Verification items for the finished model (mm, model axes). A direction names the side the tool comes from. Coordinates: 2 decimals unless noted, no trailing zeros. Order: outer loops, then holes, each group sorted by start corner. A loop starts at its lowest first (then second) coordinate and runs counter-clockwise, first axis right, second up. Notation, with made-up numbers: (55, 0) -> (112, 0) arc R26 cw to (112, 39) -> close; hole circle Ø3 at (80, 11.25). An arc over 180 degrees is marked (long way). Write item = value, one per line. Start each with the question number.
1. Go/stop test with flat-tipped pins: P1, Ø1.6, axis at x = -0.5, y = -16, coming from the +Z side; P2, Ø4, axis at x = 0, y = 0, coming from the +Z side; P3, Ø1, axis at x = -2, z = 3.5, coming from the +Y side. Record where each tip stops, or that it passes through.
2. Set-up check for faces 4 (the flat face through (-2.6, -17.5, 2.76)), 5 (the flat face through (0, -8, 4.8)), 6 (the flat face through (0, -18, 3.26)), 7 (the flat face through (-4.943, -6.509, 2.266)), 8 (the flat face through (0, -2, 2.54)): record each of +Z, -Z, +X, -X, +Y, -Y from which the full face is reachable in a straight line by a thin tool's end or side.
3. Cross-section at B-B on y = -23.5. Record the cut outline in (x, z).
4. Release check for a two-part mould opening along Y. For faces 1 (the cylindrical face through (-0.345, -1.552, 1.252)), 2 (the flat face through (-0.071, -12.448, 1.361)), 3 (the flat face through (0, -4, 0)) record: +Y half, -Y half, draft (parallel to the pull), parting line (faces both ways), or undercut.
5. Thickness scan on line 1 along X through (y, z) = (0, 2.05); line 2 along Y through (x, z) = (0, 1.45); line 3 along Y through (x, z) = (0, 0.6). Record the ranges inside material, lowest first. Write a range as from..to.
6. Cross-section at C-C on x = -3.75. Record the cut outline in (y, z).
7. Cross-section at A-A on y = 0. Record the cut outline in (x, z), plus the area to 3 significant figures.
8. Cross-section at D-D on z = 1.8. Record the cut outline in (x, y), plus the area to 3 significant figures.
from build123d import *

# Parameters (mm, degrees)
SKETCH1_W          = 10.16
SKETCH1_H          = 15.87
SKETCH1_R          = 1.59
EXTRUDE1_DEPTH     = 4.8
SKETCH2_W          = 4.533761675
SKETCH2_H          = 11.038854263
CUT_EXTRUDE1_DEPTH = 5.5
CHAMFER1_SIZE      = 1
EXTRUDE2_DEPTH     = 0.5
DRAFT1_START       = -14
DRAFT1_DEPTH       = 17.3
DRAFT1_START_2     = 3.226433484
DRAFT1_2_OUTLINE_W = 14
DRAFT1_2_OUTLINE_H = 3
DRAFT1_2_DEPTH     = 0.773566516
DRAFT2_ANGLE       = -5
DRAFT4_START       = -5.08
DRAFT4_DEPTH       = 10.16
DRAFT4_2_DEPTH     = 1.805
DRAFT4_START_2     = 3.275
DRAFT4_3_DEPTH     = 1.805
DRAFT4_START_3     = -1.805
DRAFT4_4_DEPTH     = 1.07
DRAFT4_START_4     = 0.735
DRAFT4_5_DEPTH     = 1.07
DRAFT3_ANGLE       = 5


with BuildPart() as part:
    # Sketch1 → Extrude1 (new body)
    with BuildSketch(Plane.XY):
        with Locations((0, -4.635)):
            Rectangle(SKETCH1_W, SKETCH1_H)
        Circle(SKETCH1_R, mode=Mode.SUBTRACT)
    extrude(amount=EXTRUDE1_DEPTH)

    # Sketch2 → Cut-Extrude1 (cut, symmetric)
    with BuildSketch(Plane(origin=(0, 0, 0), x_dir=(0, 0, -1), z_dir=(1, 0, 0))):
        with Locations((-4.806880837, 2.139427131)):
            Rectangle(SKETCH2_W, SKETCH2_H)
    extrude(amount=CUT_EXTRUDE1_DEPTH, both=True, mode=Mode.SUBTRACT)

    # Chamfer1
    chamfer1_edges = [part.edges().sort_by_distance(p)[0] for p in [
        (0, -3.38, 4.8),
    ]]
    chamfer(chamfer1_edges, length=CHAMFER1_SIZE)

    # Sketch3 → Extrude2 (add)
    with BuildSketch(Plane.XY.offset(2.76)):
        Polygon((0.735, -12.57), (0.735, -15.219762979), (0.4, -15.8), (0.4, -25.160288568), (0.175, -25.55), (-0.175, -25.55), (-0.4, -25.160288568), (-0.4, -15.8), (-0.735, -15.219762979), (-0.735, -12.57), align=None)
        Polygon((3.275, -12.57), (1.805, -12.57), (1.805, -15.219762979), (2.14, -15.8), (2.14, -25.160288568), (2.365, -25.55), (2.715, -25.55), (2.94, -25.160288568), (2.94, -15.8), (3.275, -15.219762979), align=None)
        Polygon((-1.805, -12.57), (-3.275, -12.57), (-3.275, -15.219762979), (-2.94, -15.8), (-2.94, -25.160288568), (-2.715, -25.55), (-2.365, -25.55), (-2.14, -25.160288568), (-2.14, -15.8), (-1.805, -15.219762979), align=None)
    extrude(amount=EXTRUDE2_DEPTH)

    # Draft1: read off the stored shape, not the designer's step
    # Draft1 outline → Draft1 (cut)
    with BuildSketch(Plane(origin=(0, 0, 0), x_dir=(1, 0, 0), z_dir=(0, 1, 0)).offset(DRAFT1_START)):
        Polygon((5.08, 0), (5.018757936, 0), (5.08, -0.7), align=None)
        Polygon((-5.08, -0.7), (-5.018757936, 0), (-5.08, 0), align=None)
    extrude(amount=DRAFT1_DEPTH, mode=Mode.SUBTRACT)

    # Draft1 2 outline → Draft1 2 (cut)
    with BuildSketch(Plane(origin=(0, 0, 0), x_dir=(1, 0, 0), z_dir=(0, 0.9961946980917455, -0.08715574274765836)).offset(DRAFT1_START_2)):
        with Locations((0, -0.5)):
            Rectangle(DRAFT1_2_OUTLINE_W, DRAFT1_2_OUTLINE_H)
    extrude(amount=DRAFT1_2_DEPTH, mode=Mode.SUBTRACT)

    # Draft2
    draft2_faces = [part.faces().sort_by_distance(p)[0] for p in [
        (5.08, -6.046569578, 2.451893477),
        (-5.08, -6.046569578, 2.451893477),
        (0, 3.3, 1.62),
    ]]
    draft(draft2_faces, Plane(origin=(0, 0, 0.7), x_dir=(-1, 0, 0), z_dir=(0, 0, -1)), DRAFT2_ANGLE)

    # Draft4: read off the stored shape, not the designer's step
    # Draft4 outline → Draft4 (cut)
    with BuildSketch(Plane.YZ.offset(DRAFT4_START)):
        Polygon((-12.526255668, 3.26), (-12.391523126, 4.8), (-12.57, 4.8), (-12.57, 3.26), align=None)
    extrude(amount=DRAFT4_DEPTH, mode=Mode.SUBTRACT)

    # Draft4 2 outline → Draft4 2 (cut)
    with BuildSketch(Plane.YZ.offset(DRAFT4_START)):
        Polygon((-12.57, 2.76), (-12.526255668, 3.26), (-12.57, 3.26), align=None)
    extrude(amount=DRAFT4_2_DEPTH, mode=Mode.SUBTRACT)

    # Draft4 3 outline → Draft4 3 (cut)
    with BuildSketch(Plane.YZ.offset(DRAFT4_START_2)):
        Polygon((-12.57, 2.76), (-12.526255668, 3.26), (-12.57, 3.26), align=None)
    extrude(amount=DRAFT4_3_DEPTH, mode=Mode.SUBTRACT)

    # Draft4 4 outline → Draft4 4 (cut)
    with BuildSketch(Plane.YZ.offset(DRAFT4_START_3)):
        Polygon((-12.57, 2.76), (-12.526255668, 3.26), (-12.57, 3.26), align=None)
    extrude(amount=DRAFT4_4_DEPTH, mode=Mode.SUBTRACT)

    # Draft4 5 outline → Draft4 5 (cut)
    with BuildSketch(Plane.YZ.offset(DRAFT4_START_4)):
        Polygon((-12.57, 2.76), (-12.526255668, 3.26), (-12.57, 3.26), align=None)
    extrude(amount=DRAFT4_5_DEPTH, mode=Mode.SUBTRACT)

    # Draft3
    draft3_faces = [part.faces().sort_by_distance(p)[0] for p in [
        (0, -12.57, 1.372462039),
    ]]
    draft(draft3_faces, Plane(origin=(0, 0, 2.76), x_dir=(-1, 0, 0), z_dir=(0, 0, -1)), DRAFT3_ANGLE)


solid = part.part
Worked out:
q1.P1 = 3.26
q1.P2 = 2.54
q1.P3 = -3.38
q2.face_4 = -Z, +X, -X, -Y
q2.face_5 = +Z, +X, -X, +Y, -Y
q2.face_6 = +Z, +X, -X, -Y
q2.face_7 = +Z, -X, +Y, -Y
q2.face_8 = +Z, +X, -X, +Y
q3.outline = (-2.94, 2.76) -> (-2.14, 2.76) -> (-2.14, 3.26) -> (-2.94, 3.26) -> close; (-0.4, 2.76) -> (0.4, 2.76) -> (0.4, 3.26) -> (-0.4, 3.26) -> close; (2.14, 2.76) -> (2.94, 2.76) -> (2.94, 3.26) -> (2.14, 3.26) -> close
q4.face_1 = undercut
q4.face_2 = -Y half
q4.face_3 = draft
q5.line_1 = -4.96..-1.59, 1.59..4.96
q5.line_2 = -12.46..-1.59, 1.59..3.23
q5.line_3 = -12.38..-1.59, 1.59..3.29
q6.outline = (-12.57, 2.76) -> (-12.33, 0) -> (3.24, 0) -> (3.3, 0.7) -> (3.14, 2.54) -> (-3.38, 2.54) -> (-3.38, 3.8) -> (-4.38, 4.8) -> (-12.39, 4.8) -> close
q7.outline = (-5.08, 0.7) -> (-5.02, 0) -> (-1.59, 0) -> (-1.59, 2.54) -> (-4.92, 2.54) -> close; (1.59, 0) -> (5.02, 0) -> (5.08, 0.7) -> (4.92, 2.54) -> (1.59, 2.54) -> close
q7.area = 17.4 mm²
q8.outline = (-4.98, -12.49) -> (4.98, -12.49) -> (4.98, 3.2) -> (-4.98, 3.2) -> close; hole circle Ø3.18 at (0, 0)
q8.area = 148 mm²
